Autodesk Inventor part; units mm, degrees
ref_plane "XZ Plane" through (0, 0, 0) normal (0, 1, 0) x (-1, 0, 0)
ref_plane "XY Plane" through (0, 0, 0) normal (0, 0, 1) x (1, 0, 0)
sketch "Sketch1" plane through (0, 0, 0) normal (0, 0, 1) x (1, 0, 0)
  line L0 (-19.05, -19.05) -> (19.05, -19.05)
  line L1 (19.05, -19.05) -> (19.05, 19.05)
  line L2 (19.05, 19.05) -> (-19.05, 19.05)
  line L3 (-19.05, 19.05) -> (-19.05, -19.05)
  line L4 (-19.05, -19.05) -> (19.05, 19.05) construction
  line L5 (19.05, -19.05) -> (-19.05, 19.05) construction
  line L6 (-15.875, -15.875) -> (15.875, -15.875)
  line L7 (15.875, -15.875) -> (15.875, 15.875)
  line L8 (15.875, 15.875) -> (-15.875, 15.875)
  line L9 (-15.875, 15.875) -> (-15.875, -15.875)
  line L10 (-15.875, -15.875) -> (15.875, 15.875) construction
  line L11 (15.875, -15.875) -> (-15.875, 15.875) construction
  point P0 (0, 0)
  dimension "d0" = 38.1
  dimension "d1" = 3.175
extrude "Extrusion1" add sketch "Sketch1" against normal blind 762
properties part number "1_5inSquareArmTube"
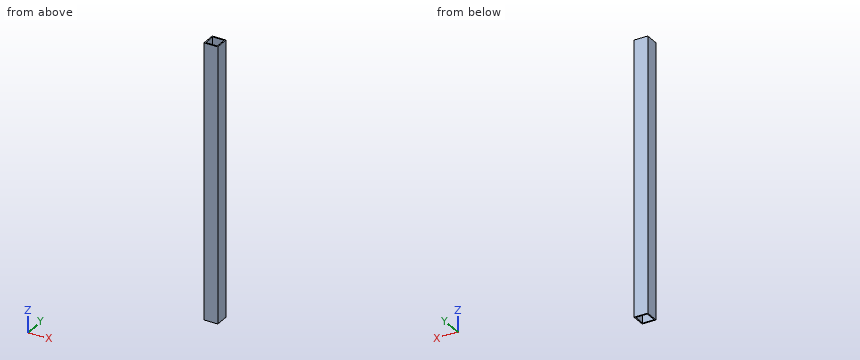
Part model, mm, in its own coordinate system. Give positions to 0.01 mm unless a question says otherwise; leave off trailing zeros. Loops run counter-clockwise (first coordinate to the right, second up) from the corner with the lowest first, then second, coordinate; pieces in that order, holes last.
(1) Band-saw the part on A-A (x = -8). Write the cut outline in (y, z) (3 decimals), and give its area (3 significant figures).
Return value:
outline: (-19.05, -762) - (-15.875, -762) - (-15.875, 0) - (-19.05, 0) - close; (15.875, -762) - (19.05, -762) - (19.05, 0) - (15.875, 0) - close
area: 4,840 mm2
(2) Drill centre line: line 1 along X through (y, z) = (5, -598) (3 decimals). Where is it in solid material? Low to high.
Return value:
line 1: x = -19.05 to -15.875, 15.875 to 19.05
(3) Band-saw the part on C-C (z = -53). Write the cut outline in (x, y) (3 decimals), and give its area (3 significant figures).
Return value:
outline: (-19.05, -19.05) - (19.05, -19.05) - (19.05, 19.05) - (-19.05, 19.05) - close; hole (-15.875, -15.875) - (15.875, -15.875) - (15.875, 15.875) - (-15.875, 15.875) - close
area: 444 mm2
